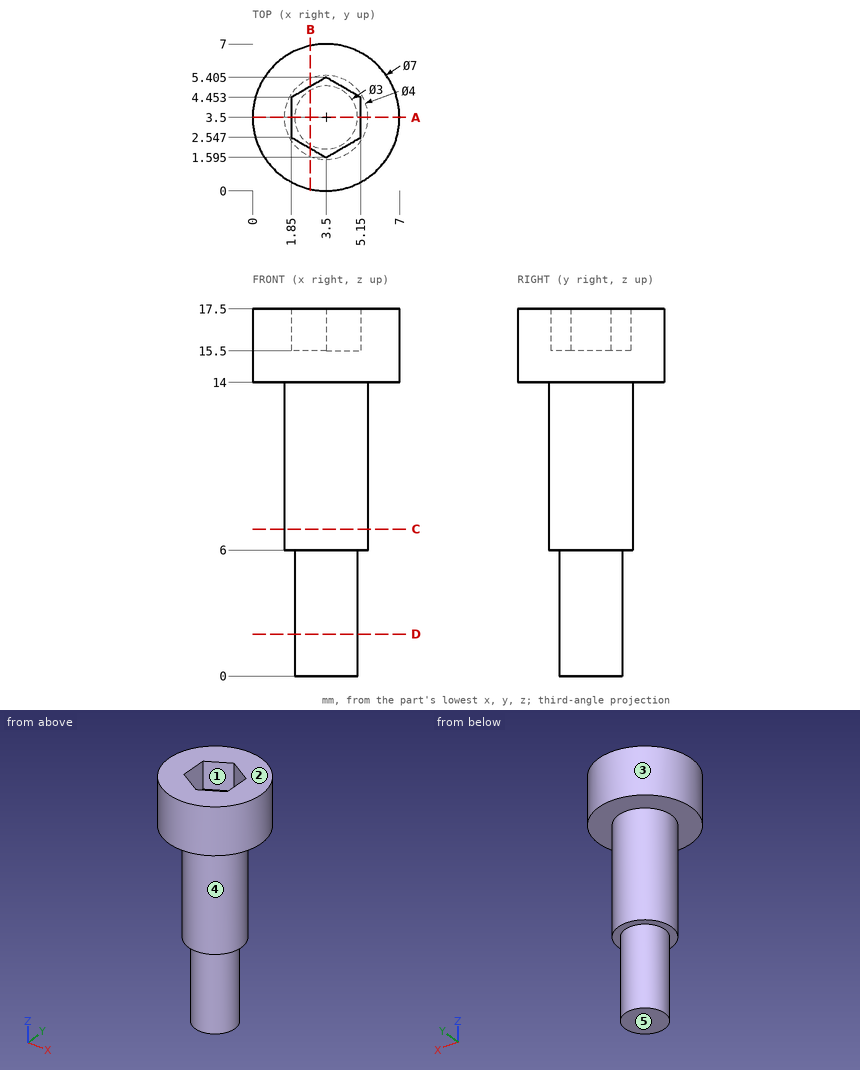
Check sheet for the drawn part. Datum: minimum x, y, z corner. Units: mm. A direction names the side the tool comes from. Give positions to 0.01 mm unless a question says otherwise; leave off trailing zeros. Order: outer loops, then holes, each group sorted by start corner. A loop starts at its lowest first (then second) coordinate and runs counter-clockwise, first axis right, second up.
1. Access from +Z, -Z, +X, -X, +Y, -Y to the whole of each face (thin tool, end or side, straight path). Record for the marked faces 4 and 5.
Completed:
face 4: -Z
face 5: -Z, +X, -X, +Y, -Y
2. Scan lines: line 1 (Z direction, x = 1, y = 3.75); line 2 (Z direction, x = 1.75, y = 4.25); line 3 (Y direction, x = 3.25, z = 8) (1 decimal). Record each from-to range of solid material in increasing order.
Completed:
line 1: z = 14 to 17.5
line 2: z = 6 to 17.5
line 3: y = 1.5 to 5.5
3. Sectioned sample at B-B (x = 2.75). Record the boundary of the cut face in (y, z), then the cut area to 3 significant figures.
Completed:
outline: (0.08, 14) - (1.65, 14) - (1.65, 6) - (2.2, 6) - (2.2, 0) - (4.8, 0) - (4.8, 6) - (5.35, 6) - (5.35, 14) - (6.92, 14) - (6.92, 17.5) - (4.97, 17.5) - (4.97, 15.5) - (2.03, 15.5) - (2.03, 17.5) - (0.08, 17.5) - close
area: 63.3 mm2
4. Depth check by flat-ended pin: pin 1 (2 mm diameter, centred on y = 3, z = 17, fed in from +X); pin 2 (1 mm diameter, centred on y = 2, z = 13, fed in from -X); pin 3 (1 mm diameter, centred on x = 3, y = 3, fed in from +Z); pin 4 (1.5 mm diameter, centred on x = 3, z = 11, fed in from +Y). Enter the tip coordinate at first touch or a pass-through.
Completed:
pin 1: stops at x = 7
pin 2: stops at x = 1.77
pin 3: stops at z = 15.5
pin 4: stops at y = 5.5
5. Sectioned sample at A-A (y = 3.5). Record the boundary of the cut face in (x, z), then the cut area to 3 significant figures.
Completed:
outline: (0, 14) - (1.5, 14) - (1.5, 6) - (2, 6) - (2, 0) - (5, 0) - (5, 6) - (5.5, 6) - (5.5, 14) - (7, 14) - (7, 17.5) - (5.15, 17.5) - (5.15, 15.5) - (1.85, 15.5) - (1.85, 17.5) - (0, 17.5) - close
area: 67.9 mm2
6. Sectioned sample at C-C (z = 7). Record the boundary of the cut face in (x, y).
Completed:
outline: circle Ø4 at (3.5, 3.5)
7. Sectioned sample at D-D (z = 2). Record the boundary of the cut face in (x, y).
Completed:
outline: circle Ø3 at (3.5, 3.5)
8. Draft check along X on the marked faces 1, 2 and 3. Enter one of: pulls with the +X half, pulls with the -X half, needs draft (parallel to the pull), parting line crosses it, or undercut.
Completed:
face 1: undercut
face 2: needs draft
face 3: parting line crosses it
